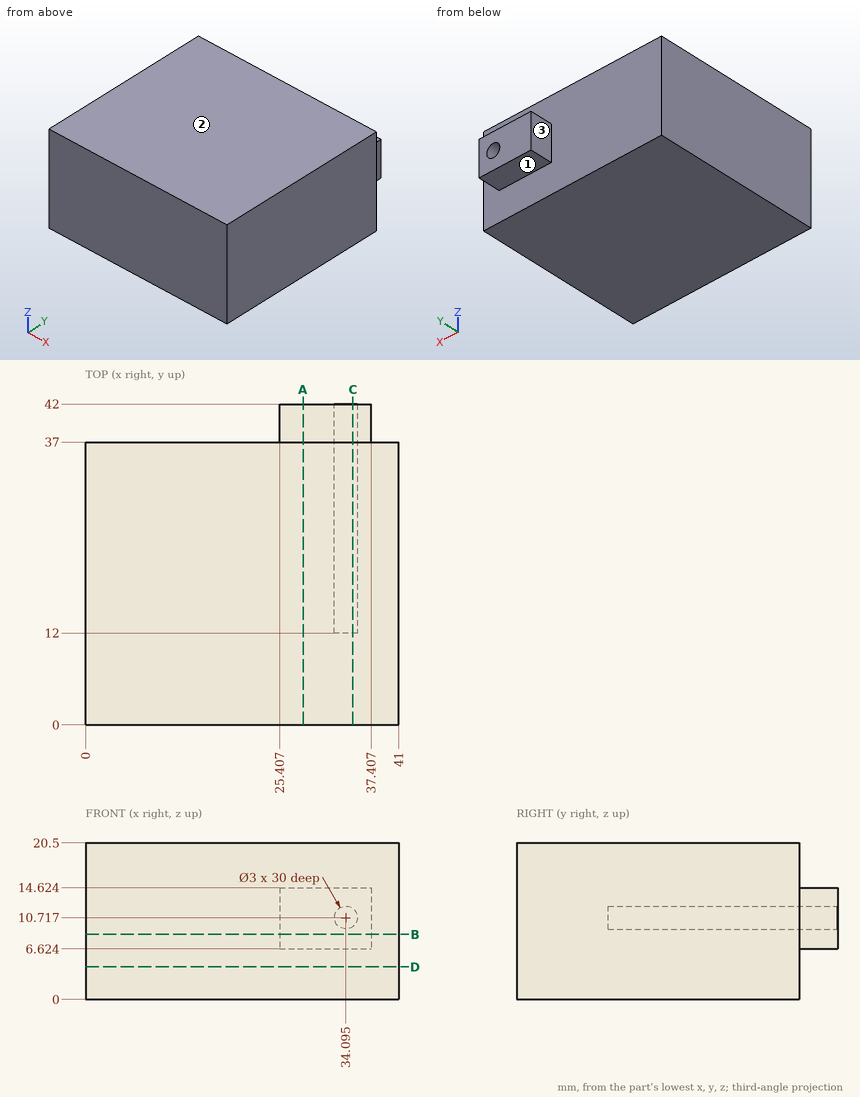
Design review of the part shown in the three views and the two pictorial views. Dimensions are in mm from the part's minimum x, y and z. A direction names the side the tool comes from. Coordinates: 2 decimals unless noted, no trailing zeros. Order: outer loops, then holes, each group sorted by start corner. A loop starts at its lowest first (then second) coordinate and runs counter-clockwise, first axis right, second up.
1) Wall thickness on line 1 along Y through (x, z) = (29.5, 19.75); line 2 along X through (y, z) = (28, 10.5); line 3 along X through (y, z) = (33.5, 11.5) (1 decimal): over which ranges is each line inside the solid? List them lowest first.
2) Take a section at C-C, the plane x = 35. Give the boundary of the cut face in (y, z), and give its area (3 significant figures).
3) Take a section at A-A, the plane x = 28.5. Give the boundary of the cut face in (y, z).
4) Clearance check with flat-ended pins moving along their axes: pin 1 (2.5 mm diameter, centred on x = 34.1, z = 10.72, fed in from +Y); pin 2 (1.5 mm diameter, centred on y = 39.5, z = 11.5, fed in from +X); pin 3 (4 mm diameter, centred on x = 14.5, z = 2.5, fed in from +Y). State where each tip first meets the part, or that it passes through.
5) Take a section at B-B, the plane z = 8.5. Give the boundary of the cut face in (x, y).
6) Take a section at D-D, the plane z = 4.25. Give the boundary of the cut face in (x, y).
7) For the marked faces 1, 2 and 3, list the 3-axis set-ups (+Z, -Z, +X, -X, +Y, -Y) from which the entire face can be reached by the end or side of a thin tool; tool diameter is ignored.
Returned:
1. line 1: y = 0 to 37
1. line 2: x = 0 to 32.61, 35.58 to 41
1. line 3: x = 0 to 32.8, 35.4 to 41
2. outline: (0, 0) - (37, 0) - (37, 6.62) - (42, 6.62) - (42, 9.52) - (12, 9.52) - (12, 11.91) - (42, 11.91) - (42, 14.62) - (37, 14.62) - (37, 20.5) - (0, 20.5) - close
2. area: 727 mm2
3. outline: (0, 0) - (37, 0) - (37, 6.62) - (42, 6.62) - (42, 14.62) - (37, 14.62) - (37, 20.5) - (0, 20.5) - close
4. pin 1: stops at y = 12
4. pin 2: stops at x = 37.41
4. pin 3: stops at y = 37
5. outline: (0, 0) - (41, 0) - (41, 37) - (37.41, 37) - (37.41, 42) - (25.41, 42) - (25.41, 37) - (0, 37) - close
6. outline: (0, 0) - (41, 0) - (41, 37) - (0, 37) - close
7. face 1: -Z, +X, -X, +Y
7. face 2: +Z, +X, -X, +Y, -Y
7. face 3: +Z, -Z, -X, +Y
